Here's the drawing with two shaded views (mm, measured from the low corner). I have some questions. A direction names the side the tool comes from. Round coordinates to 2 decimals unless told otherwise and drop trailing zeros. Loops run counter-clockwise (first coordinate to the right, second up) from the corner with the lowest first, then second, coordinate; pieces in that order, holes last.
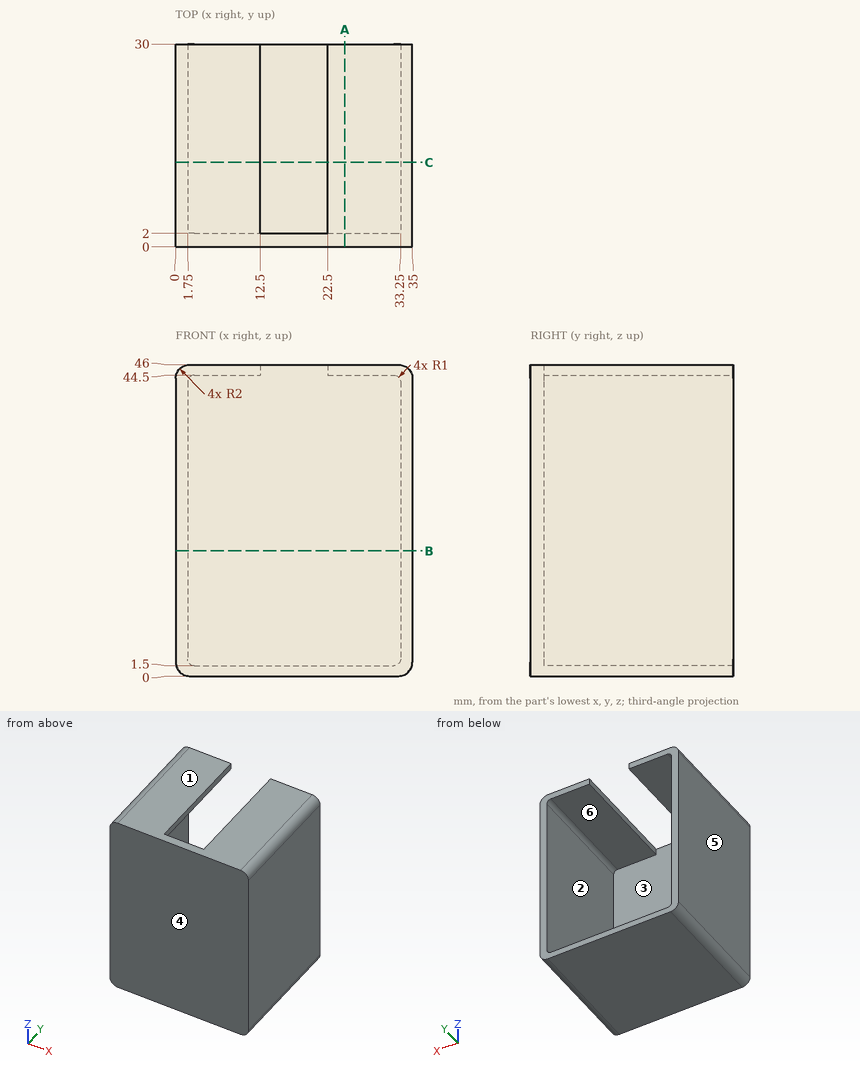
Item 1: If we section it at B-B, the plane z = 18.5: Please give me the cut outline in (x, y).
Results list:
outline: (0, 0) - (35, 0) - (35, 30) - (33.25, 30) - (33.25, 2) - (1.75, 2) - (1.75, 30) - (0, 30) - close
Item 2: If we section it at C-C, the plane y = 12.5: Please give me the cut outline in (x, z), then the cut area to 3 significant figures.
Results list:
outline: (0, 2) arc R2 ccw to (2, 0) - (33, 0) arc R2 ccw to (35, 2) - (35, 44) arc R2 ccw to (33, 46) - (22.5, 46) - (22.5, 44.5) - (32.25, 44.5) arc R1 cw to (33.25, 43.5) - (33.25, 2.5) arc R1 cw to (32.25, 1.5) - (2.75, 1.5) arc R1 cw to (1.75, 2.5) - (1.75, 43.5) arc R1 cw to (2.75, 44.5) - (12.5, 44.5) - (12.5, 46) - (2, 46) arc R2 ccw to (0, 44) - close
area: 238 mm2
Item 3: We'd pull the mould along X, two halves only. Please class the marked faces 3, 4, 5 and 6: released by +X, released by -X, zero draft, split by the parting line, or undercut.
Results list:
face 3: undercut
face 4: zero draft
face 5: released by -X
face 6: undercut
Item 4: For the marked faces 1 and 2, which set-ups out of +Z, -Z, +X, -X, +Y, -Y let a thin tool reach every point of the face, with its end or its side?
Results list:
face 1: +Z, +X, -X, +Y, -Y
face 2: +Y
Item 5: If we section it at A-A, the plane x = 25: Please give me the cut outline in (y, z).
Results list:
outline: (0, 0) - (30, 0) - (30, 1.5) - (2, 1.5) - (2, 44.5) - (30, 44.5) - (30, 46) - (0, 46) - close
Item 6: If I drill on line 1 along X through (y, z) = (27.5, 13.5); line 2 along Z through (x, y) = (24.5, 15.25); line 3 along Y through (x, z) = (11, 24.5), over which ranges is the centre line in solid material (lowest first)?
Results list:
line 1: x = 0 to 1.75, 33.25 to 35
line 2: z = 0 to 1.5, 44.5 to 46
line 3: y = 0 to 2
Item 7: Will these pins go through, and if not, where does the flat tip stop? pin 1 (1 mm diameter, centred on x = 23, z = 14.5, fed in from -Y); pin 2 (16 mm diameter, centred on x = 11, z = 18, fed in from +Y); pin 3 (4 mm diameter, centred on x = 16, y = 17, fed in from +Z); pin 4 (1.2 mm diameter, centred on y = 16.5, z = 45.5, fed in from +X).
Results list:
pin 1: stops at y = 0
pin 2: stops at y = 2
pin 3: stops at z = 1.5
pin 4: stops at x = 34.79
